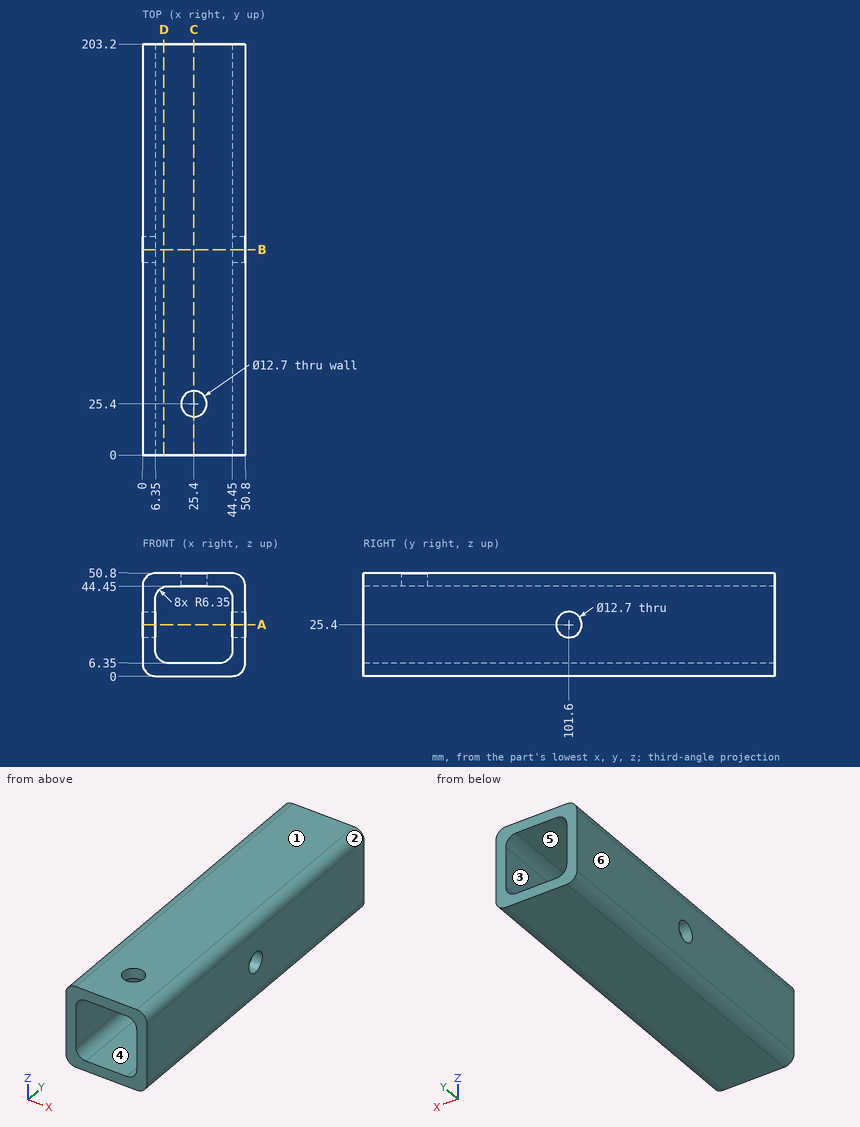
Source: three-view drawing plus pictorial views. Frame: mm from the lowest corner of the part. A direction names the side the tool comes from. Coordinates: 2 decimals unless noted, no trailing zeros. Order: outer loops, then holes, each group sorted by start corner. A loop starts at its lowest first (then second) coordinate and runs counter-clockwise, first axis right, second up. Notation, with made-up numbers: M 50.25,40.5 L 81.25,40.5 A24 ccw 81.25,76.5 Z; hole C 23.5,-24.75 d2. An arc over 180 degrees is marked long. Answer in a Markdown table with one row per item.
(1) Section query C-C, the plane x = 25.4. Output: boundary loops of the cut face in (y, z).
Numbers:
| item | result |
|---|---|
| outline | M 0,0 L 203.2,0 L 203.2,6.35 L 0,6.35 Z; M 0,44.45 L 19.05,44.45 L 19.05,50.8 L 0,50.8 Z; M 31.75,44.45 L 203.2,44.45 L 203.2,50.8 L 31.75,50.8 Z |
(2) Section query A-A, the plane z = 25.4. Output: boundary loops of the cut face in (x, y).
Numbers:
| item | result |
|---|---|
| outline | M 0,0 L 6.35,0 L 6.35,95.25 L 0,95.25 Z; M 0,107.95 L 6.35,107.95 L 6.35,203.2 L 0,203.2 Z; M 44.45,0 L 50.8,0 L 50.8,95.25 L 44.45,95.25 Z; M 44.45,107.95 L 50.8,107.95 L 50.8,203.2 L 44.45,203.2 Z |
(3) Section query B-B, the plane y = 101.6. Output: boundary loops of the cut face in (x, z), plus the area to 3 significant figures.
Numbers:
| item | result |
|---|---|
| outline | M 0,6.35 A6.35 ccw 6.35,0 L 44.45,0 A6.35 ccw 50.8,6.35 L 50.8,19.05 L 44.45,19.05 L 44.45,12.7 A6.35 cw 38.1,6.35 L 12.7,6.35 A6.35 cw 6.35,12.7 L 6.35,19.05 L 0,19.05 Z; M 0,31.75 L 6.35,31.75 L 6.35,38.1 A6.35 cw 12.7,44.45 L 38.1,44.45 A6.35 cw 44.45,38.1 L 44.45,31.75 L 50.8,31.75 L 50.8,44.45 A6.35 ccw 44.45,50.8 L 6.35,50.8 A6.35 ccw 0,44.45 Z |
| area | 968 mm^2 |
(4) Access query for the marked faces 5 and 6. Directions: +Z, -Z, +X, -X, +Y, -Y. A direction counts if a zero-diameter tool reaches every point of the face in a straight line with its end or side. Return the directions, or none.
Numbers:
| item | result |
|---|---|
| face 5 | +Y, -Y |
| face 6 | +Z, -Z, -X, +Y, -Y |
(5) Material intervals for line 1 (Z direction, x = 35, y = 60); line 2 (Y direction, x = 25.4, z = 48.25), sorted ascending. Write a range as [from, to].
Numbers:
| item | result |
|---|---|
| line 1 | z = [0, 6.35], [44.45, 50.8] |
| line 2 | y = [0, 19.05], [31.75, 203.2] |
(6) Section query D-D, the plane x = 10.5. Output: boundary loops of the cut face in (y, z), plus the area to 3 significant figures.
Numbers:
| item | result |
|---|---|
| outline | M 0,0 L 203.2,0 L 203.2,6.74 L 0,6.74 Z; M 0,44.06 L 203.2,44.06 L 203.2,50.8 L 0,50.8 Z |
| area | 2,740 mm^2 |
(7) Draft query along X for the marked faces 1, 2, 3 and 4. Return one class per face: pulls with the +X half, pulls with the -X half, needs draft (parallel to the pull), parting line crosses it, or undercut.
Numbers:
| item | result |
|---|---|
| face 1 | needs draft |
| face 2 | pulls with the +X half |
| face 3 | undercut |
| face 4 | undercut |
